Autodesk Inventor part; units mm, degrees
ref_plane "Work Plane1" through (0, 7, 0) normal (0, 1, 0) x (1, 0, 0)
ref_plane "YZ Plane" through (0, 0, 0) normal (1, 0, 0) x (0, 1, 0)
ref_plane "XZ Plane" through (0, 0, 0) normal (0, 1, 0) x (-1, 0, 0)
sketch "Sketch1" plane through (0, 0, 0) normal (0, 1, 0) x (-1, 0, 0)
  line L0 (7.3724, 5.1622) -> (14.7447, 0)
  line L1 (14.7447, 0) -> (7.3724, -5.1622)
  line L2 (0.5606, 8.9825) -> (9.1932, 11.5279)
  line L3 (9.1932, 11.5279) -> (8.6326, 2.5454)
  line L4 (-6.6733, 6.0388) -> (-3.281, 14.3751)
  line L5 (-3.281, 14.3751) -> (3.3923, 8.3362)
  line L6 (-8.8821, -1.4522) -> (-13.2845, 6.3975)
  line L7 (-13.2845, 6.3975) -> (-4.4025, 7.8497)
  line L8 (-4.4025, -7.8497) -> (-13.2845, -6.3975)
  line L9 (-13.2845, -6.3975) -> (-8.8821, 1.4522)
  line L10 (3.3923, -8.3362) -> (-3.281, -14.3751)
  line L11 (-3.281, -14.3751) -> (-6.6733, -6.0388)
  line L12 (8.6326, -2.5454) -> (9.1932, -11.5279)
  line L13 (9.1932, -11.5279) -> (0.5606, -8.9825)
  arc A0 (-6.6733, -6.0388) -> (-5.3444, -7.2414) centre (0, 0) ccw
  arc A1 (7.3724, -5.1622) -> (7.957, -4.2054) centre (0, 0) ccw
  arc A2 (8.2491, -3.599) -> (8.6326, -2.5454) centre (0, 0) ccw
  point P0 (-6.0457, -7.5811)
  point P1 (2.1577, -9.4534)
  point P2 (8.7363, -4.2072)
  point P3 (8.7363, 4.2072)
  point P4 (2.1577, 9.4534)
  point P5 (-6.0457, 7.5811)
  point P6 (-9.6965, 0)
  dimension "d5" = 360
extrude "Extrusion1" add sketch "Sketch1" along normal blind 2
sketch "Sketch2" plane through (0, 2, 0) normal (0, 1, 0) x (1, 0, 0)
  circle A0 centre (0, 0) radius 4.5
  dimension "d9" = 9
extrude "Extrusion2" add sketch "Sketch2" along normal blind 14
sketch "Sketch3" plane through (0, 16, 0) normal (0, 1, 0) x (1, 0, 0)
  arc A0 (-1.976, -1.6898) -> (-1.976, 1.6898) centre (0, 0) ccw
  line L0 (-1.976, -1.6898) -> (-1.976, 1.6898)
  line L1 (2.6, 0) -> (2.6, 18.1631)
  dimension "d19" = 2.6
extrude "Extrusion3" cut sketch "Sketch3" against normal through all
sketch "Sketch4" plane through (-1.976, 16, 1.6898) normal (1, 0, 0) x (0, 0, -1)
  circle A0 centre (1.6248, -3.7675) radius 1.425
  point P0 (1.6898, -16)
  dimension "d16" = 2.85
extrude "Extrusion4" cut sketch "Sketch4" against normal blind 10
sketch "Sketch5" plane through (0, 0, 0) normal (0, -1, 0) x (1, 0, 0)
  circle A0 centre (0, 0) radius 4.5
  line L0 (-1.976, -1.6898) -> (-1.976, 1.6898)
  line L1 (-1.976, 1.6898) -> (-1.976, -1.6898)
  arc A1 (-1.976, -1.6898) -> (-1.976, 1.6898) centre (0, 0) ccw
  dimension "d20" = 9
extrude "Extrusion5" add sketch "Sketch5" along normal blind 5
sketch "Sketch6" plane through (0, -5, 0) normal (0, -1, 0) x (1, 0, 0)
  arc A0 (-1.976, -1.6898) -> (-1.976, 1.6898) centre (0, 0) ccw
  circle A1 centre (0, 0) radius 14.5
  point P0 (0, 0)
  dimension "d23" = 29
extrude "Extrusion6" add sketch "Sketch6" along normal blind 3
ref_plane "Work Plane1" through (0, 7, 0) normal (0, 1, 0) x (1, 0, 0)
sketch "Sketch7" plane through (0, 7, 0) normal (0, 1, 0) x (1, 0, 0)
  circle A0 centre (0, 0) radius 4.5
  arc A1 (-1.976, -1.6898) -> (-1.976, 1.6898) centre (0, 0) ccw
  circle A2 centre (0, 0) radius 14.5
extrude "Extrusion7" add sketch "Sketch7" along normal blind 3
properties part number "gear"
Work out the finished part from the listing and answer in its coordinate system (mm). A direction names the side the tool comes from. Give positions to 0.01 mm unless a question says otherwise; leave off trailing zeros. Order: outer loops, then holes, each group sorted by start corner. A loop starts at its lowest first (then second) coordinate and runs counter-clockwise, first axis right, second up. Notation, with made-up numbers: (89, -3.75) - (148, -3.75) arc R19 cw to (148, 9.25) - close; hole circle Ø9 at (22, 41). An arc over 180 degrees is marked (long way). One line per item, written item: value. Start each with the question number.
1. For a pull along Y with two mould halves and no side action, classify faces 1 (the face through (0, -8, 0)), 2 (the face through (2, 16, 2)), 3 (the face through (11.516, 0.986, -3.244)) as released by +Y, released by -Y, zero draft, split by the parting line, or undercut.
2. Which of the six approach directions +Z, -Z, +X, -X, +Y, -Y give full straight-line access (tool end or side, diameter ignored) to faces 4 (the face through (0.524, 0.986, -11.88)), 5 (the face through (9.72, 0.99, 6.98)), 6 (the face through (-8.96, 0.99, -7.82))?
3. Consider line 1 (Y direction, x = -12, z = 1); line 2 (Z direction, x = 0, y = 3.5); line 3 (Y direction, x = -7.5, z = -12.25). Determine where each line is inside the solid, lowest interval first.
4. Section D-D, the plane y = 4 is taken. Write down the section's boundary in (x, z), then the cut area to 3 significant figures.
5. Section B-B, the plane x = 5.5 is taken. Write down the section's boundary in (y, z).
6. Each of these flat-tipped pins is pushed along its axis until it touches: pin 1 Ø8.5 at (x, z) = (-2.5, -7) entering from +Y; pin 2 Ø1.4 at (x, z) = (0, 0) entering from +Y; pin 3 Ø4 at (y, z) = (9.5, -11) entering from -X; pin 4 Ø3.5 at (y, z) = (2.5, -0.5) entering from +X. Where does it stop, or does it pass through?
7. Section C-C, the plane z = 8.25 is taken. Write down the section's boundary in (x, y), then the cut area to 3 significant figures.
Filled sheet:
1. face 1: released by -Y
1. face 2: released by +Y
1. face 3: undercut
2. face 4: -Z
2. face 5: +Z, +X
2. face 6: -X
3. line 1: -8 to -5, 0 to 2, 7 to 10
3. line 2: -4.5 to -2.6, 2.6 to 4.5
3. line 3: -8 to -5, 7 to 10
4. outline: circle Ø9 at (0, 0); hole (-1.98, -1.69) arc R2.6 ccw (long way) to (-1.98, 1.69) - close
4. area: 43.8 mm²
5. outline: (-8, -13.42) - (-5, -13.42) - (-5, 13.42) - (-8, 13.42) - close; (0, -8.92) - (2, -8.92) - (2, 8.92) - (0, 8.92) - close; (7, -13.42) - (10, -13.42) - (10, 13.42) - (7, 13.42) - close
6. pin 1: y = 16
6. pin 2: y = -5
6. pin 3: x = -11.37
6. pin 4: x = 10.92
7. outline: (-11.92, -8) - (11.92, -8) - (11.92, -5) - (-11.92, -5) - close; (-11.92, 7) - (11.92, 7) - (11.92, 10) - (-11.92, 10) - close; (-8.99, 0) - (5.77, 0) - (5.77, 2) - (-8.99, 2) - close
7. area: 173 mm²
